CAD build for the part. Positions are in the model's coordinates, mm. A direction names the side the tool comes from. Round coordinates to 2 decimals unless told otherwise and drop trailing zeros. Write each loop counter-clockwise with the first axis right and the second up, starting at its lowest first coordinate (ties: lowest second). Pieces come first, ordered by that corner, then holes. Notation, with made-up numbers: (72, -36) - (87, -36) arc R35 cw to (87, 2) - close; hole circle Ø7 at (-21, -30.75). An arc over 180 degrees is marked (long way). Put each result on its own line as item: value. Start each with the question number.
Item 1: Cut at A-A (x = -28.6). Count the separate pieces of the cut face and the enclosed holes in it, and give its area (3 significant figures).
Item 2: Cut at C-C (z = 27.5). Give the cut face in (x, y).
Item 3: Pin check, flat tips, straight feed: pin 1 Ø5 at (x, y) = (-27, 7.5) entering from +Z; pin 2 Ø4.5 at (y, z) = (38, 26.5) entering from -X. Stop position of each tip, or through.
Item 4: 3-axis set-ups, long thin cutter, end or side, ignore diameter. For faces 1 (the cylindrical face through (-31.19, 66.73, 14.62)), 2 (the cylindrical face through (-33.557, 6.651, 31.938)): which of +Z, -Z, +X, -X, +Y, -Y reach the whole face in a straight line?
Item 5: Drill centre lines: line 1 (Y direction, x = -28.6, z = 30.45); line 2 (X direction, y = 6, z = 21.5); line 3 (Y direction, x = -28.6, z = 10.5). Where is each one in solid material? Low to high. Write a range as from..to.
Item 6: Cut at B-B (y = 67.3). Give the cut face in (x, z), and give its area (3 significant figures).
Item 7: Cut at D-D (y = 36.65). Give the cut face in (x, z), and give its area (3 significant figures).
Item 8: Mould opens along Y. For faces 3 (the flat face through (-18, 73.3, 17)), 4 (the flat face through (-17, 0, 17)), 5 (the cylindrical face through (-31.96, 32.26, 26.52)), 6 (the flat face through (-34.6, 36, 17)) say: released by +Y, released by -Y, zero draft, split by the parting line, or undercut.
Autodesk Inventor part; units mm, degrees
ref_plane "YZ Plane" through (0, 0, 0) normal (1, 0, 0) x (0, 1, 0)
ref_plane "XZ Plane" through (0, 0, 0) normal (0, 1, 0) x (-1, 0, 0)
ref_plane "XY Plane" through (0, 0, 0) normal (0, 0, 1) x (1, 0, 0)
sketch "Sketch5" plane through (0, 0, 0) normal (0, 0, 1) x (1, 0, 0)
  line L0 (0, 0) -> (-34.6, 0)
  line L1 (-34.6, 0) -> (-34.6, 73.3)
  line L2 (-34.6, 73.3) -> (0, 73.3)
  line L3 (0, 73.3) -> (0, 0)
  dimension "d7" = 34.6
  dimension "d8" = 73.3
sketch "Sketch6" plane through (0, 0, 0) normal (0, 0, 1) x (1, 0, 0)
  point P0 (0, 0)
extrude "Extrusion3" add sketch "Sketch5" along normal blind 35
sketch "Sketch7" plane through (0, 0, 35) normal (0, 0, 1) x (1, 0, 0)
  line L0 (-34.6, 0) -> (0, 0)
  line L1 (-34.6, 0) -> (-34.6, 6)
  line L2 (-34.6, 73.3) -> (-34.6, 0)
  line L3 (-34.6, 6) -> (-28.6, 6)
  dimension "d11" = 6
  dimension "d12" = 6
hole "Hole1" at (-28.6, 6, 35) direction (0, 0, -1) diameter 5.3 end through all counterbore diameter 10 counterbore depth 5.7
ref_plane "Work Plane1" through (-34.6, 36.65, 0) normal (0, 1, 0) x (1, 0, 0)
mirror "Mirror1" about plane through (-34.6, 36.65, 0) normal (0, 1, 0) of "Hole1"
sketch "Sketch8" plane through (-34.6, 0, 0) normal (-1, 0, 0) x (0, 0, 1)
  point P0 (0, 0)
sketch "Sketch9" plane through (-34.6, 0, 0) normal (-1, 0, 0) x (0, 0, 1)
  line L0 (0, 0) -> (35, 0)
  line L1 (0, 0) -> (0, 36.65)
  line L2 (0, 73.3) -> (0, 0)
  line L3 (0, 36.65) -> (27.5, 36.65)
  circle A0 centre (27.5, 36.65) radius 4.5
  dimension "d20" = 36.65
  dimension "d21" = 27.5
  dimension "d22" = 9
extrude "Extrusion4" cut sketch "Sketch9" against normal blind 5
fillet "Fillet1" radius 0.5 12 edges at (0, 73.3, 17.5) (-34.6, 73.3, 17.5) (0, 0, 17.5) (-34.6, 0, 17.5) (-17.3, 0, 35) (-17.3, 0, 0) (0, 36.65, 0) (-34.6, 36.65, 0) (-17.3, 73.3, 0) (-17.3, 73.3, 35) (0, 36.65, 35) (-34.6, 36.65, 35)
chamfer "Chamfer1" distance 0.35 angle 45 1 edges at (-28.6, 11, 35)
chamfer "Chamfer2" distance 0.35 angle 45 1 edges at (-28.6, 62.3, 35)
chamfer "Chamfer3" distance 0.35 angle 45 2 edges at (-28.6, 8.65, 0) (-28.6, 64.65, 0)
chamfer "Chamfer4" distance 0.35 angle 45 1 edges at (-34.6, 36.65, 23)
properties part number "springHolder"
Output values:
1. separate pieces: 3
1. enclosed holes: 0
1. area: 2,140 mm2
2. outline: (-34.6, 0.5) arc R0.5 ccw to (-34.1, 0) - (-0.5, 0) arc R0.5 ccw to (0, 0.5) - (0, 72.8) arc R0.5 ccw to (-0.5, 73.3) - (-34.1, 73.3) arc R0.5 ccw to (-34.6, 72.8) - (-34.6, 41.5) - (-34.25, 41.15) - (-29.6, 41.15) - (-29.6, 32.15) - (-34.25, 32.15) - (-34.6, 31.8) - close; hole circle Ø5.3 at (-28.6, 6); hole circle Ø5.3 at (-28.6, 67.3)
3. pin 1: z = 29.3
3. pin 2: x = -29.6
4. face 1: +Z, -Z
4. face 2: +Z
5. line 1: 0..1, 11..62.3, 72.3..73.3
5. line 2: -34.6..-31.25, -25.95..0
5. line 3: 0..3.35, 8.65..64.65, 69.95..73.3
6. outline: (-34.6, 0.5) arc R0.5 ccw to (-34.1, 0) - (-31.6, 0) - (-31.25, 0.35) - (-31.25, 29.3) - (-33.6, 29.3) - (-33.6, 34.65) - (-33.95, 35) - (-34.1, 35) arc R0.5 ccw to (-34.6, 34.5) - close; (-25.95, 0.35) - (-25.6, 0) - (-0.5, 0) arc R0.5 ccw to (0, 0.5) - (0, 34.5) arc R0.5 ccw to (-0.5, 35) - (-23.25, 35) - (-23.6, 34.65) - (-23.6, 29.3) - (-25.95, 29.3) - close
6. area: 998 mm2
7. outline: (-34.6, 0.5) arc R0.5 ccw to (-34.1, 0) - (-0.5, 0) arc R0.5 ccw to (0, 0.5) - (0, 34.5) arc R0.5 ccw to (-0.5, 35) - (-34.1, 35) arc R0.5 ccw to (-34.6, 34.5) - (-34.6, 32.35) - (-34.25, 32) - (-29.6, 32) - (-29.6, 23) - (-34.25, 23) - (-34.6, 22.65) - close
7. area: 1,170 mm2
8. face 3: released by +Y
8. face 4: released by -Y
8. face 5: undercut
8. face 6: zero draft
